```python
from build123d import *

# Parameters (mm, degrees)
F1_DEPTH = 3


with BuildPart() as f1:
    # F0 (on Front) → F1 (new body)
    with BuildSketch(Plane.XZ):
        with BuildLine():
            Line((33.051588, 17.876159), (30.149128, 23.294637))
            ThreePointArc((30.149128, 23.294637), (-36.690424, -10.26756), (37.860809, -4.262528))
            Line((37.860809, -4.262528), (33.393364, -4.506392))
            ThreePointArc((33.393364, -4.506392), (33.384315, -4.572946), (33.375133, -4.639482))
            ThreePointArc((33.375133, -4.639482), (-10.299233, -32.083487), (-29.839553, 15.653286))
            Line((-29.839553, 15.653286), (0, -31.200437))
            Line((0, -31.200437), (33.051588, 17.876159))
        make_face()
        with BuildLine():
            Line((0, -23.174103), (-26.297564, 18.11803))
            ThreePointArc((-26.297564, 18.11803), (-0.009919, 31.880483), (26.034596, 17.663288))
            Line((26.034596, 17.663288), (0, -23.174103))
        make_face(mode=Mode.SUBTRACT)
    extrude(amount=F1_DEPTH)


solid = f1.part
```
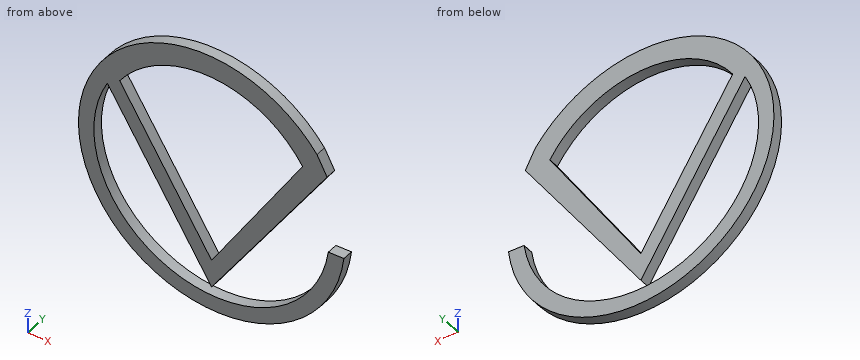
Build history of the part. All positions in model axes, mm. Coordinates: 2 decimals unless noted, no trailing zeros. Write each loop counter-clockwise with the first axis right and the second up, starting at its lowest first coordinate (ties: lowest second). Pieces come first, ordered by that corner, then holes.
1. Drop flat-ended pins along their axis: pin 1 (1.5 mm diameter, centred on x = -18, y = -2, fed in from +Z); pin 2 (1.5 mm diameter, centred on x = 22.5, z = 7, fed in from +Y); pin 3 (1 mm diameter, centred on x = 24.5, y = -1.5, fed in from +Z); pin 4 (1.5 mm diameter, centred on y = -1.5, z = -16, fed in from +X). Give the stop position or say it passes through.
Answer block:
pin 1: stops at z = 33.97
pin 2: stops at y = 0
pin 3: stops at z = 29.59
pin 4: stops at x = 34.91
2. Band-saw the part on C-C, the plane x = 4. Give the cut face in (y, z).
Answer block:
outline: (-3, -37.89) - (0, -37.89) - (0, -33.46) - (-3, -33.46) - close; (-3, -25.26) - (0, -25.26) - (0, -16.9) - (-3, -16.9) - close; (-3, 31.59) - (0, 31.59) - (0, 37.89) - (-3, 37.89) - close
3. Band-saw the part on D-D, the plane z = -7.5. Give the cut face in (x, y), and give its area (3 significant figures).
Answer block:
outline: (-37.35, -3) - (-32.85, -3) - (-32.85, 0) - (-37.35, 0) - close; (-15.09, -3) - (-9.98, -3) - (-9.98, 0) - (-15.09, 0) - close; (9.99, -3) - (15.96, -3) - (15.96, 0) - (9.99, 0) - close; (32.85, -3) - (37.35, -3) - (37.35, 0) - (32.85, 0) - close
area: 60.3 mm2
4. Band-saw the part on A-A, the plane y = -1.1. Give the cut face in (x, z), and give its area (3 significant figures).
Answer block:
outline: (-29.84, 15.65) - (0, -31.2) - (33.05, 17.88) - (30.15, 23.29) arc R38.1 ccw (long way) to (37.86, -4.26) - (33.39, -4.51) arc R33.61 cw to (33.38, -4.64) arc R33.7 cw (long way) to start; hole (-26.3, 18.12) - (0, -23.17) - (26.03, 17.66) arc R31.47 ccw to start
area: 1,510 mm2
5. Drill centre lines: probe 1 along Z at (x, y) = (1, -0.35); probe 2 along X at (y, z) = (-0.9, -24); probe 3 along Z at (x, y) = (0.5, -0.6). Where is each one in solid material? Low to high.
Answer block:
probe 1: z = -38.09 to -33.68, -29.72 to -21.61, 31.86 to 38.09
probe 2: x = -29.59 to -23.65, -4.59 to 4.85, 23.65 to 29.59
probe 3: z = -38.1 to -33.69, -30.46 to -22.39, 31.87 to 38.1
6. Band-saw the part on B-B, the plane z = 2.5. Give the cut face in (x, y), and give its area (3 significant figures).
Answer block:
outline: (-38.02, -3) - (-33.6, -3) - (-33.6, 0) - (-38.02, 0) - close; (-21.46, -3) - (-16.35, -3) - (-16.35, 0) - (-21.46, 0) - close; (16.37, -3) - (22.7, -3) - (22.7, 0) - (16.37, 0) - close
area: 47.6 mm2
